Part model, mm, in its own coordinate system. A direction names the side the tool comes from. Round coordinates to 2 decimals unless told otherwise and drop trailing zeros. Order: outer loops, then holes, each group sorted by start corner. A loop starts at its lowest first (then second) coordinate and runs counter-clockwise, first axis right, second up. Notation, with made-up numbers: (62, 15) - (117, 15) arc R25 ccw to (117, 33) - close; hole circle Ø9 at (-30.75, 16). An arc over 180 degrees is marked (long way). Answer as a JSON object with one key per item and string values.
Autodesk Inventor part; units mm, degrees
ref_plane "YZ Plane" through (0, 0, 0) normal (1, 0, 0) x (0, 1, 0)
ref_plane "XZ Plane" through (0, 0, 0) normal (0, 1, 0) x (-1, 0, 0)
ref_plane "XY Plane" through (0, 0, 0) normal (0, 0, 1) x (1, 0, 0)
sketch "Sketch1" plane through (0, 0, 0) normal (0, 1, 0) x (-1, 0, 0)
  line L0 (6.7, 6.7) -> (-6.7, 6.7)
  line L1 (-6.7, 6.7) -> (-6.7, -6.7)
  line L2 (-6.7, -6.7) -> (6.7, -6.7)
  line L3 (6.7, -6.7) -> (6.7, 6.7)
  point P0 (0, 0)
  dimension "d0" = 13.4
  dimension "d1" = 13.4
  dimension "d2" = 6.7
  dimension "d3" = 6.7
extrude "Extrusion1" add sketch "Sketch1" along normal blind 2
sketch "Sketch2" plane through (0, 0, 0) normal (0, -1, 0) x (1, 0, 0)
  line L0 (6.7, 6.7) -> (6.7, -6.7)
  line L1 (6.7, 6.7) -> (6.7, -6.7)
  line L2 (-6.7, -6.7) -> (-6.7, 6.7)
  line L3 (6.7, -6.7) -> (-6.7, -6.7)
  line L4 (-6.7, -6.7) -> (-6.7, 6.7)
  line L5 (-6.7, 6.7) -> (6.7, 6.7)
  line L6 (4.7, 4.7) -> (-4.7, 4.7)
  line L7 (-4.7, 4.7) -> (-4.7, -4.7)
  line L8 (-4.7, -4.7) -> (4.7, -4.7)
  line L9 (4.7, -4.7) -> (4.7, 4.7)
  line L10 (4.7, -2) -> (6.7, -2)
  line L11 (6.7, 2) -> (4.7, 2)
  point P0 (0, 0)
  point P1 (0, 4.7)
  point P2 (5.7, 2)
  point P3 (4.7, 0)
  dimension "d6" = 2
  dimension "d8" = 2
  dimension "d9" = 2
  dimension "d10" = 2
  dimension "d11" = 4
  dimension "d12" = 2
extrude "Extrusion2" cut sketch "Sketch2" against normal blind 2 contours L0 L10 L9 L11
sketch "Sketch3" plane through (0, 0, 0) normal (0, -1, 0) x (1, 0, 0)
  line L0 (-6.7, -6.7) -> (-6.7, 6.7)
  line L1 (-6.7, 2) -> (-4.7, 2)
  line L2 (-4.7, 2) -> (-4.7, -2)
  line L3 (-4.7, -2) -> (-6.7, -2)
  point P0 (0, 0)
  point P1 (-6.7, 0)
  dimension "d15" = 2
  dimension "d16" = 2
  dimension "d17" = 4
extrude "Extrusion3" cut sketch "Sketch3" against normal blind 1
sketch "Sketch4" plane through (4.7, 0, 2) normal (1, 0, 0) x (0, 0, -1)
  line L0 (0, 2) -> (4, 2)
  line L1 (4, 0) -> (4, 1)
  line L2 (0, 2) -> (4, 2)
  line L3 (4, 2) -> (4, 1)
  line L4 (4, 1) -> (0, 1)
  line L5 (0, 1) -> (0, 2)
  point P0 (2, 0)
extrude "Extrusion4" add sketch "Sketch4" along normal blind 2
sketch "Sketch5" plane through (0, 0, 0) normal (0, -1, 0) x (1, 0, 0)
  line L0 (6.7, 6.7) -> (6.7, 2)
  line L1 (-6.7, 2) -> (-6.7, 6.7)
  line L2 (6.7, 2.15) -> (-6.7, 2.15)
  line L3 (-6.7, 2.15) -> (-6.7, -2.15)
  line L4 (-6.7, -2.15) -> (6.7, -2.15)
  line L5 (6.7, -2.15) -> (6.7, 2.15)
  line L6 (-4.7, -2) -> (-6.7, -2)
  point P0 (0, 0)
  point P1 (-6.7, 2.15)
  dimension "d22" = 4.3
  dimension "d23" = 0.15
extrude "Extrusion5" cut sketch "Sketch5" against normal blind 1
sketch "Sketch6" plane through (0, 1, 0) normal (0, -1, 0) x (1, 0, 0)
  line L0 (6.7, 6.7) -> (6.7, -6.7)
  line L1 (-6.7, 2) -> (6.7, 2)
  line L2 (6.7, 2) -> (6.7, -2)
  line L3 (6.7, -2) -> (-6.7, -2)
  line L4 (-6.7, -2) -> (-6.7, 2)
  line L5 (-6.7, 2.15) -> (6.7, 2.15)
  line L6 (6.7, -2.15) -> (-6.7, -2.15)
  line L7 (6.7, -2) -> (6.7, -2.15)
  line L8 (6.7, -2.15) -> (-6.7, -2.15)
  line L9 (-6.7, -2) -> (-6.7, -2.15)
  line L10 (-6.7, 2) -> (-6.7, 2.15)
  line L11 (-6.7, 2.15) -> (6.7, 2.15)
  line L12 (6.7, 2.15) -> (6.7, 2)
  point P0 (0, 0)
  dimension "d26" = 0.15
  dimension "d27" = 0.15
  dimension "d28" = 13.4
extrude "Extrusion6" add sketch "Sketch6" along normal blind 1 contours L0 L1 L10 L5 | L0 L6 L9 L3
properties part number "Camera_Housing_Top"
Item 1: Cut at A-A (y = 0.2). Write the cut outline in (x, z).
Taken from the geometry:
{"outline": "(-6.7, -6.7) - (6.7, -6.7) - (6.7, -2) - (-6.7, -2) - close; (-6.7, 2) - (6.7, 2) - (6.7, 6.7) - (-6.7, 6.7) - close"}
Item 2: Probe L1, parallel to Z at x = 5, y = 0.6; L2, parallel to Y at x = -2, z = 0. List the from-to ranges inside material, lowest first. Write a range as from..to.
Taken from the geometry:
{"L1": "-6.7..-2, 2..6.7", "L2": "1..2"}
Item 3: Drop flat-ended pins along their axis: P1, Ø6, axis at x = 0, z = -2.5, coming from the -Y side; P2, Ø1.2, axis at x = 2, z = -0.5, coming from the -Y side. Give the stop position or say it passes through.
Taken from the geometry:
{"P1": "y = 0", "P2": "y = 1"}
Item 4: Cut at C-C (z = -0.5). Write the cut outline in (x, y).
Taken from the geometry:
{"outline": "(-6.7, 1) - (6.7, 1) - (6.7, 2) - (-6.7, 2) - close"}
Item 5: Two-plate mould, pull along Z, no slides. Class faces 3 (the flat face through (-0.1, 0.5, 2)), 4 (the flat face through (0, 0, -4)), 5 (the flat face through (0, 1, 0)), 6 (the flat face through (0, 1, 6.7)): pulls with the +Z half, pulls with the -Z half, needs draft (parallel to the pull), parting line crosses it, or undercut.
Taken from the geometry:
{"face 3": "undercut", "face 4": "needs draft", "face 5": "undercut", "face 6": "pulls with the +Z half"}
Item 6: Tool access for faces 1 (the flat face through (0.1, 0.5, -2)), 2 (the flat face through (0, 1, -6.7)): list every direction of +Z, -Z, +X, -X, +Y, -Y with a clear straight run to the whole face (end or side of a thin tool).
Taken from the geometry:
{"face 1": "+X, -X, -Y", "face 2": "-Z, +X, -X, +Y, -Y"}
Item 7: Cut at B-B (x = -5.5). Write the cut outline in (y, z).
Taken from the geometry:
{"outline": "(0, -6.7) - (2, -6.7) - (2, 6.7) - (0, 6.7) - (0, 2) - (1, 2) - (1, -2) - (0, -2) - close"}
